Geometry: final body of the model. Coordinates: model frame, mm. A direction names the side the tool comes from. Round coordinates to 2 decimals unless told otherwise and drop trailing zeros. Write each loop counter-clockwise with the first axis right and the second up, starting at its lowest first coordinate (ties: lowest second). Pieces come first, ordered by that corner, then holes. Notation, with made-up numbers: M 42,39 L 90,39 A21 ccw 90,78 Z; hole C 83.5,-25 d6. An arc over 180 degrees is marked long. Put each result on its own line as item: value. Start each with the question number.
```python
from build123d import *

# Parameters (mm, degrees)
SKETCH_2_R          = 8
EXTRUDE_1_DEPTH     = 22.9
SKETCH_4_R          = 10.68097998
EXTRUDE_3_DEPTH     = 2
CHAMFER_1_SIZE      = 0.5
CHAMFER_1_SIZE2     = 1.37373871
CHAMFER_2_SIZE      = 0.5
CHAMFER_2_SIZE2     = 1.37373871
CUT_EXTRUDE_1_DEPTH = 2
SKETCH_9_W          = 0.6
SKETCH_9_H          = 8


with BuildPart() as part:
    # 草图2 → 凸台-拉伸1 (new body)
    with BuildSketch(Plane(origin=(0, 0, 0), x_dir=(1, 0, 0), z_dir=(0, 1, 0))):
        with Locations(Location((0, 0, 0), (0, 0, 270))):
            Circle(SKETCH_2_R)
    extrude(amount=EXTRUDE_1_DEPTH)

    # 草图4 → 凸台-拉伸3 (add)
    with BuildSketch(Plane.XZ):
        with Locations(Location((0, 0, 0), (0, 0, 270))):
            Circle(SKETCH_4_R)
    extrude(amount=-EXTRUDE_3_DEPTH)

    # 倒角1
    chamfer_1_edges = [part.edges().sort_by_distance(p)[0] for p in [
        (0, 0, 10.68097998),
    ]]
    chamfer_1_side = [part.faces().sort_by_distance(p)[0] for p in [
        (0, 1, 10.68097998),
    ]]
    chamfer(chamfer_1_edges, length=CHAMFER_1_SIZE, length2=CHAMFER_1_SIZE2, reference=chamfer_1_side[0])

    # 倒角2
    chamfer_2_edges = [part.edges().sort_by_distance(p)[0] for p in [
        (0, 2, 10.68097998),
    ]]
    chamfer_2_side = [part.faces().sort_by_distance(p)[0] for p in [
        (0, 1.25, 10.68097998),
    ]]
    chamfer(chamfer_2_edges, length=CHAMFER_2_SIZE, length2=CHAMFER_2_SIZE2, reference=chamfer_2_side[0])

    # 草图1 → 切除-拉伸1 (cut)
    with BuildSketch(Plane(origin=(0, 0, 0), x_dir=(1, 0, 0), z_dir=(0, 1, 0))):
        with BuildLine():
            Line((5.34048999, 9.25), (10.68097998, 0))
            ThreePointArc((10.68097998, 0), (9.25, 5.34048999), (5.34048999, 9.25))
        make_face()
        with BuildLine():
            Line((-5.34048999, 9.25), (5.34048999, 9.25))
            ThreePointArc((5.34048999, 9.25), (0, 10.68097998), (-5.34048999, 9.25))
        make_face()
        with BuildLine():
            ThreePointArc((5.34048999, -9.25), (9.25, -5.34048999), (10.68097998, 0))
            Line((10.68097998, 0), (5.34048999, -9.25))
        make_face()
        with BuildLine():
            ThreePointArc((-5.34048999, -9.25), (0, -10.68097998), (5.34048999, -9.25))
            Line((5.34048999, -9.25), (-5.34048999, -9.25))
        make_face()
        with BuildLine():
            ThreePointArc((-10.68097998, 0), (-9.25, -5.34048999), (-5.34048999, -9.25))
            Line((-5.34048999, -9.25), (-10.68097998, 0))
        make_face()
        with BuildLine():
            Line((-10.68097998, 0), (-5.34048999, 9.25))
            ThreePointArc((-5.34048999, 9.25), (-9.25, 5.34048999), (-10.68097998, 0))
        make_face()
    extrude(amount=CUT_EXTRUDE_1_DEPTH, mode=Mode.SUBTRACT)

    # 草图6 → 旋转1 (revolve)
    with BuildSketch(Plane.XY, mode=Mode.PRIVATE) as revolve_1_sk:
        with BuildLine():
            Line((0, 0), (9, 0))
            ThreePointArc((9, 0), (9.4, -0.4), (9, -0.8))
            Line((9, -0.8), (0, -0.8))
            Line((0, -0.8), (0, 0))
        make_face()
    revolve(revolve_1_sk.sketch.rotate(Axis((0, 0, 0), (0, -1, 0)), 270), axis=Axis((0, 0, 0), (0, -1, 0)))

    # 草图7 → 旋转2 (revolve)
    with BuildSketch(Plane.XY, mode=Mode.PRIVATE) as revolve_2_sk:
        with BuildLine():
            Line((0, -0.8), (10.6, -0.8))
            ThreePointArc((10.6, -0.8), (10.69701425, -0.875746437), (10.647058824, -0.988235294))
            Line((10.647058824, -0.988235294), (8.441176471, -2.164705882))
            ThreePointArc((8.441176471, -2.164705882), (7.98507125, -2.340285), (7.5, -2.4))
            Line((7.5, -2.4), (0, -2.4))
            Line((0, -2.4), (0, -0.8))
        make_face()
    revolve(revolve_2_sk.sketch.rotate(Axis((0, -2.4, 0), (0, 1, 0)), 90), axis=Axis((0, -2.4, 0), (0, 1, 0)))

    # 草图9 → 切除-旋转1 (revolve, cut)
    with BuildSketch(Plane.XY, mode=Mode.PRIVATE) as cut_revolve_1_sk:
        with Locations((7.7, 18.9)):
            Rectangle(SKETCH_9_W, SKETCH_9_H)
    revolve(cut_revolve_1_sk.sketch.rotate(Axis((0, 0, 0), (0, 1, 0)), 90), axis=Axis((0, 0, 0), (0, 1, 0)), mode=Mode.SUBTRACT)

    # 草图10 → 旋转4 (revolve)
    with BuildSketch(Plane.XY, mode=Mode.PRIVATE) as revolve_4_sk:
        Polygon((4.153927956, 22.9), (4.653927956, 22.9), (4.653927956, 24.9), (5.353927956, 24.9), (5.353927956, 25.9), (4.153927956, 25.9), align=None)
    revolve_4 = revolve(revolve_4_sk.sketch.rotate(Axis((4.153927956, 22.9, 0), (0, 1, 0)), 90), axis=Axis((4.153927956, 22.9, 0), (0, 1, 0)))

    # 镜向1: 旋转4 across plane
    add(revolve_4.mirror(Plane(origin=(0, 0, 0), x_dir=(0, 0, 1), z_dir=(1, 0, 0))))


solid = part.part
```
1) Section A-A, the plane x = 0. Output: boundary loops of the cut face in (y, z), and give its area (3 significant figures).
2) First-contact query: pin 1 (2 mm diameter, centred on y = 14, z = 6, fed in from -X) (3 decimals); pin 2 (12 mm diameter, centred on x = 3, y = 19.5, fed in from -Z); pin 3 (1 mm diameter, centred on x = -1, y = 0.5, fed in from -Z). Flat tips, straight axial feed; report the tip coordinate or a pass-through.
3) Section C-C, the plane y = 19.5. Output: boundary loops of the cut face in (x, z), and give its area (3 significant figures).
4) Access query for faces 1 (the face through (-4.888, 0.135, -8.354)), 2 (the face through (6, 14.9, 5)), 3 (the face through (8.05, 0.99, 4.56)), 4 (the face through (0, 1, 9.25)). Directions: +Z, -Z, +X, -X, +Y, -Y. A direction counts if a zero-diameter tool reaches every point of the face in a straight line with its end or side. Return the directions, or none.
5) Ray query, probe 1 along Y at (x, z) = (6.25, 3.75); probe 2 along X at (y, z) = (21.25, 0); probe 3 along Z at (x, y) = (0.5, 16.75). Return the intervals inside material, ascending.
6) Draft query along X for faces 5 (the face through (5, 24.9, 0)), 6 (the face through (-7.973, 0.986, 4.69)), 7 (the face through (4.888, 1.865, 8.354)). Return one class per face: +X half, -X half, draft (parallel to the pull), parting line (faces both ways), or undercut.
7) Section B-B, the plane y = 14.25. Output: boundary loops of the cut face in (x, z).
Solved:
1. outline: M -2.4,-7.5 A2 ccw -2.16,-8.44 L -0.99,-10.65 A0.1 ccw -0.8,-10.6 L -0.8,-9 A0.4 ccw 0,-9 L 0,-9.25 L 2,-9.25 L 2,-8 L 14.9,-8 L 14.9,-7.4 L 22.9,-7.4 L 22.9,7.4 L 14.9,7.4 L 14.9,8 L 2,8 L 2,9.25 L 0,9.25 L 0,9 A0.4 ccw -0.8,9 L -0.8,10.6 A0.1 ccw -0.99,10.65 L -2.16,8.44 A2 ccw -2.4,7.5 Z
1. area: 407 mm2
2. pin 1: stops at x = -6.245
2. pin 2: stops at z = -8
2. pin 3: stops at z = -9.25
3. outline: C 0,0 d14.8
3. area: 172 mm2
4. face 1: -Z, -X
4. face 2: +Y
4. face 3: +Z, +X, +Y
4. face 4: +Z, +X, -X, +Y
5. probe 1: y = -2.4 to 22.9
5. probe 2: x = -7.4 to 7.4
5. probe 3: z = -7.38 to 7.38
6. face 5: undercut
6. face 6: -X half
6. face 7: +X half
7. outline: C 0,0 d16
